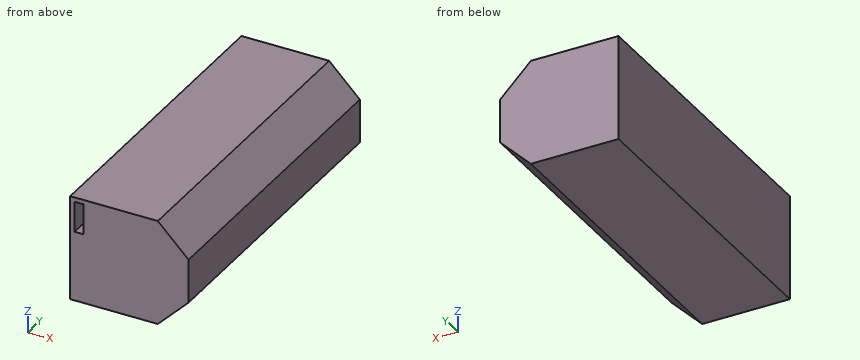
Autodesk Fusion 360 part; units mm, degrees
sketch "Sketch1" plane through (0, 0, 0) normal (1, 0, 0) x (0, 1, 0) in component "RobotisBatt"
  line L0 (0, 0) -> (71, 0)
  line L1 (71, 0) -> (71, 24)
  line L2 (71, 24) -> (0, 24)
  line L3 (0, 24) -> (0, 0)
  dimension "d1" = 71
  dimension "d2" = 24
extrude "Extrude1" add sketch "Sketch1" along normal blind 27 in component "RobotisBatt"
chamfer "Chamfer1" distance 7 angle 45 2 edges at (27, 35.5, 24) (27, 35.5, 0) in component "RobotisBatt"
sketch "Sketch2" plane through (0, 0, 0) normal (0, -1, 0) x (1, 0, 0) in component "RobotisBatt"
  line L0 (20, 0) -> (27, 7)
  line L1 (27, 7) -> (27, 17)
  line L2 (27, 17) -> (20, 24)
  line L3 (20, 24) -> (0, 24)
  line L4 (0, 24) -> (0, 0)
  line L5 (0, 0) -> (20, 0)
  line L6 (1, 23) -> (3, 23)
  line L7 (3, 23) -> (3, 16)
  line L8 (3, 16) -> (1, 16)
  line L9 (1, 16) -> (1, 23)
extrude "Extrude2" cut sketch "Sketch2" against normal blind 4 contours L6 L7 L8 L9 in component "RobotisBatt"
component "RobotisBatt" placed x (1, 0, 0) y (0, 1, 0) z (0, 0, 1) at (0, 0, 0)
The listing builds one solid part. Answer for the finished solid, in the listing's coordinates (mm). Coordinates: 2 decimals unless noted, no trailing zeros. Write each loop counter-clockwise with the first axis right and the second up, starting at its lowest first coordinate (ties: lowest second). Pieces come first, ordered by that corner, then holes. Notation, with made-up numbers: (2.5, -37) - (48.5, -37) arc R17 cw to (48.5, -8) - close; hole circle Ø1 at (33.25, 37). An arc over 180 degrees is marked (long way). Return JSON: item names as keys, results as strings. Group by question number.
Q1. Find the intervals of material crossed by line 1 along X through (y, z) = (7, 4); line 2 along X through (y, z) = (61.5, 6.5); line 3 along Z through (x, y) = (22.25, 51), in increasing order. Write a range as [from, to].
Q2. The part is cut by section C-C on z = 21. Write down the section's boundary in (x, y).
Q3. The part is cut by section D-D on z = 3.5. Write down the section's boundary in (x, y).
Q4. The part is cut by section B-B on y = 52. Write down the section's boundary in (x, z).
Q5. Flat-ended cylindrical pins translate along their axes: pin 1 Ø2 at (y, z) = (2, 20.5) entering from +X; pin 2 Ø4 at (y, z) = (32, 20.5) entering from +X. Find the tip coordinate at first contact, or state that the pin passes through.
Q6. The part is cut by section A-A on z = 17.75. Write down the section's boundary in (x, y), and give its area (3 significant figures).
Evaluation:
{
 "1": {"line 1": "x = [0, 24]", "line 2": "x = [0, 26.5]", "line 3": "z = [2.25, 21.75]"},
 "2": {"outline": "(0, 0) - (1, 0) - (1, 4) - (3, 4) - (3, 0) - (23, 0) - (23, 71) - (0, 71) - close"},
 "3": {"outline": "(0, 0) - (23.5, 0) - (23.5, 71) - (0, 71) - close"},
 "4": {"outline": "(0, 0) - (20, 0) - (27, 7) - (27, 17) - (20, 24) - (0, 24) - close"},
 "5": {"pin 1": "stops at x = 24.5", "pin 2": "stops at x = 25.5"},
 "6": {"outline": "(0, 0) - (1, 0) - (1, 4) - (3, 4) - (3, 0) - (26.25, 0) - (26.25, 71) - (0, 71) - close", "area": "1,860 mm2"}
}
